The listing builds one solid part. Answer for the finished solid, in the listing's coordinates (mm). Give positions to 0.01 mm unless a question says otherwise; leave off trailing zeros. Write each loop counter-clockwise with the first axis right and the second up, starting at its lowest first coordinate (ties: lowest second). Pieces come first, ordered by that corner, then holes. Notation, with made-up numbers: M -9.75,-21 L 35.25,-21 A19 cw 35.25,-8 Z; hole C 30.5,-12 d2. An arc over 180 degrees is marked long. Return JSON: item names as keys, results as strings.
from build123d import *

# Parameters (mm, degrees)
F0_W     = 30
F0_H     = 31
F0_R     = 3.75
F1_DEPTH = 1.25
F2_R     = 5


with BuildPart() as f1:
    # F0 (on Front) → F1 (new body, symmetric)
    with BuildSketch(Plane.XZ):
        Rectangle(F0_W, F0_H)
        Circle(F0_R, mode=Mode.SUBTRACT)
    extrude(amount=F1_DEPTH, both=True)

    # F2
    f2_edges = [f1.edges().sort_by_distance(p)[0] for p in [
        (15, 0, 15.5),
        (15, 0, -15.5),
        (-15, 0, 15.5),
        (-15, 0, -15.5),
    ]]
    fillet(f2_edges, radius=F2_R)


solid = f1.part
Item 1: Find the intervals of material crossed by line 1 (Z direction, x = 0, y = 0.05); line 2 (X direction, y = 0.2, z = 0.5); line 3 (X direction, y = -0.4, z = 13), in increasing order.
Geometry results:
{"line 1": "z = -15.5 to -3.75, 3.75 to 15.5", "line 2": "x = -15 to -3.72, 3.72 to 15", "line 3": "x = -14.33 to 14.33"}
Item 2: Given pin 1 Ø4.5 at (x, z) = (0, 0) entering from +Y; pin 2 Ø1.5 at (x, y) = (12, 0.5) entering from -Z, each flat-ended and moving along its own axis, determine where each tip first touches the part or whether it passes through.
Geometry results:
{"pin 1": "passes through", "pin 2": "stops at z = -15.34"}
Item 3: A cutting plane is placed at B-B, the plane z = 0. Write down the section's boundary in (x, y), plus the area to 4 significant figures.
Geometry results:
{"outline": "M -15,-1.25 L -3.75,-1.25 L -3.75,1.25 L -15,1.25 Z; M 3.75,-1.25 L 15,-1.25 L 15,1.25 L 3.75,1.25 Z", "area": "56.25 mm2"}
Item 4: A cutting plane is placed at D-D, the plane z = 12.5. Write down the section's boundary in (x, y), plus the area to 3 significant figures.
Geometry results:
{"outline": "M -14.58,-1.25 L 14.58,-1.25 L 14.58,1.25 L -14.58,1.25 Z", "area": "72.9 mm2"}
Item 5: Determine the mould class of faces 1 (the flat face through (-4, -1.25, 4)), 2 (the flat face through (-15, 0, 0)), 3 (the cylindrical face through (-3.746, 0.018, 0.165)), 4 (the flat face through (15, 0, 0)) for opening direction X: +X half, -X half, draft (parallel to the pull), parting line (faces both ways), or undercut.
Geometry results:
{"face 1": "draft", "face 2": "-X half", "face 3": "undercut", "face 4": "+X half"}
Item 6: A cutting plane is placed at A-A, the plane x = 0. Write down the section's boundary in (y, z), plus the area to 4 significant figures.
Geometry results:
{"outline": "M -1.25,-15.5 L 1.25,-15.5 L 1.25,-3.75 L -1.25,-3.75 Z; M -1.25,3.75 L 1.25,3.75 L 1.25,15.5 L -1.25,15.5 Z", "area": "58.75 mm2"}
Item 7: A cutting plane is placed at C-C, the plane y = 0.85. Write down the section's boundary in (x, z).
Geometry results:
{"outline": "M -15,-10.5 A5 ccw -10,-15.5 L 10,-15.5 A5 ccw 15,-10.5 L 15,10.5 A5 ccw 10,15.5 L -10,15.5 A5 ccw -15,10.5 Z; hole C 0,0 d7.5"}
